Autodesk Inventor part; units mm, degrees
ref_plane "YZ Plane" through (0, 0, 0) normal (1, 0, 0) x (0, 1, 0)
ref_plane "XZ Plane" through (0, 0, 0) normal (0, 1, 0) x (-1, 0, 0)
ref_plane "XY Plane" through (0, 0, 0) normal (0, 0, 1) x (1, 0, 0)
sketch "Sketch1" plane through (0, 0, 0) normal (0, 0, 1) x (1, 0, 0)
  circle A0 centre (0, 0) radius 2
  circle A1 centre (0, 0) radius 3.5
  circle A2 centre (0, 0) radius 1.9
  dimension "d0" = 3.8
extrude "Extrusion1" add sketch "Sketch1" against normal blind 5 and the other way blind 0.5 contours A2
sketch "Sketch2" plane through (0, 0, 0.5) normal (0, 0, 1) x (1, 0, 0)
  circle A0 centre (0, 0) radius 1.9
  circle A1 centre (0, 0) radius 3
  dimension "d3" = 6
extrude "Extrusion2" add sketch "Sketch2" along normal blind 12 contours A0 | A1
sketch "Sketch3" plane through (0, 0, 12.5) normal (0, 0, 1) x (1, 0, 0)
  circle A0 centre (0, 0) radius 3
  line L0 (-2.5981, -1.5) -> (2.5981, -1.5)
  dimension "d8" = 4.5
extrude "Extrusion3" cut sketch "Sketch3" against normal blind 10 contours L0 A0 picked at (-0.7274, -1.6862)
chamfer "Chamfer1" distance 0.5 angle 45 2 edges at (2.8978, -0.7765, 12.5) (-0.7765, 2.8978, 12.5)
properties part number "12mm Incremental Encoder Shaft"
Geometry check sheet. Reference: the model listing, model coordinates, mm. A direction names the side the tool comes from. Coordinates: 2 decimals unless noted, no trailing zeros. Loops run counter-clockwise (first coordinate to the right, second up) from the corner with the lowest first, then second, coordinate; pieces in that order, holes last. Notation, with made-up numbers: (80, -16.5) -> (99, -16.5) arc R21 cw to (99, -11.5) -> close; hole circle Ø9 at (-13.5, 48). An arc over 180 degrees is marked (long way). Put each result on its own line as item: value.
1) Cross-section at C-C on z = -2. Record the boundary of the cut face in (x, y).
Result set:
outline: circle Ø3.8 at (0, 0)
2) Thickness scan on line 1 (Y direction, x = -0.1, z = -0.75); line 2 (Z direction, x = 0.05, y = -2.6); line 3 (Y direction, x = 1.05, z = 5.5). Record the ranges inside material, lowest first.
Result set:
line 1: y = -1.9 to 1.9
line 2: z = 0.5 to 2.5
line 3: y = -1.5 to 2.81
3) Cross-section at D-D on z = 2.75. Record the boundary of the cut face in (x, y).
Result set:
outline: (-2.6, -1.5) -> (2.6, -1.5) arc R3 ccw (long way) to start
4) Tool access check on faces 1 (the conical face through (-0.08, 2.64, 12.36)), 2 (the cylindrical face through (-1.9, 0.08, -2.21)), 3 (the flat face through (0, -1.5, 8)). Record the directions out of +Z, -Z, +X, -X, +Y, -Y that give a thin tool (end or side, any length) a straight path to the whole face; none if there is none.
Result set:
face 1: +Z
face 2: -Z
face 3: +Z, +X, -X, -Y
5) Cross-section at B-B on y = 0. Record the boundary of the cut face in (x, z), plus the area to 4 significant figures.
Result set:
outline: (-3, 0.5) -> (-1.9, 0.5) -> (-1.9, -5) -> (1.9, -5) -> (1.9, 0.5) -> (3, 0.5) -> (3, 12) -> (2.5, 12.5) -> (-2.5, 12.5) -> (-3, 12) -> close
area: 92.65 mm^2
6) Gauge pin test, flat ends, axial feed: pin 1 Ø2 at (x, z) = (-2.5, 3.5) entering from +Y; pin 2 Ø1.6 at (x, z) = (0.5, 6.5) entering from -Y; pin 3 Ø1.5 at (x, y) = (-2.5, 1) entering from -Z; pin 4 Ø2 at (x, z) = (1, 1) entering from -Y. Record the tip position at first contact, or that the pin passes through.
Result set:
pin 1: stops at y = 2.6
pin 2: stops at y = -1.5
pin 3: stops at z = 0.5
pin 4: stops at y = -3
7) Cross-section at A-A on x = 0. Record the boundary of the cut face in (y, z), plus the area to 3 significant figures.
Result set:
outline: (-3, 0.5) -> (-1.9, 0.5) -> (-1.9, -5) -> (1.9, -5) -> (1.9, 0.5) -> (3, 0.5) -> (3, 12) -> (2.5, 12.5) -> (-1.5, 12.5) -> (-1.5, 2.5) -> (-3, 2.5) -> close
area: 77.8 mm^2
